from build123d import *

# Parameters (mm, degrees)
SKETCH1_W                                       = 59.1
SKETCH1_H                                       = 59.1
SKETCH1_R                                       = 19.5
SKETCH1_R_2                                     = 1.55
BOSS_EXTRUDE1_DEPTH                             = 4
SKETCH2_W                                       = 59.1
SKETCH2_H                                       = 50
SKETCH2_R                                       = 1.5
BOSS_EXTRUDE2_DEPTH                             = 4
CSK_FOR_M3_FLAT_HEAD_MACHINE_SCREW1_D           = 3.4
CSK_FOR_M3_FLAT_HEAD_MACHINE_SCREW1_CSINK_D     = 6.3
CSK_FOR_M3_FLAT_HEAD_MACHINE_SCREW1_CSINK_ANGLE = 90
CSK_FOR_M4_FLAT_HEAD_MACHINE_SCREW1_D           = 4.5
CSK_FOR_M4_FLAT_HEAD_MACHINE_SCREW1_CSINK_D     = 9.4
CSK_FOR_M4_FLAT_HEAD_MACHINE_SCREW1_CSINK_ANGLE = 90


with BuildPart() as part:
    # Sketch1 → Boss-Extrude1 (new body)
    with BuildSketch(Plane.XY):
        with Locations((23.55, 23.55)):
            Rectangle(SKETCH1_W, SKETCH1_H)
        with Locations((23.55, 23.55)):
            Circle(SKETCH1_R, mode=Mode.SUBTRACT)
        with Locations((0, 47.1)):
            Circle(SKETCH1_R_2, mode=Mode.SUBTRACT)
        with Locations((47.1, 47.1)):
            Circle(SKETCH1_R_2, mode=Mode.SUBTRACT)
        with Locations((47.1, 0)):
            Circle(SKETCH1_R_2, mode=Mode.SUBTRACT)
        Circle(SKETCH1_R_2, mode=Mode.SUBTRACT)
    extrude(amount=BOSS_EXTRUDE1_DEPTH)

    # Sketch2 → Boss-Extrude2 (add)
    with BuildSketch(Plane.XZ.offset(6)):
        with Locations((23.55, -21)):
            Rectangle(SKETCH2_W, SKETCH2_H)
        with Locations(Location((0, -40, 0), (0, 0, 270))):
            Circle(SKETCH2_R, mode=Mode.SUBTRACT)
        with Locations(Location((47.1, -40, 0), (0, 0, 270))):
            Circle(SKETCH2_R, mode=Mode.SUBTRACT)
        with Locations(Location((23.55, -18, 0), (0, 0, 270))):
            Circle(SKETCH2_R, mode=Mode.SUBTRACT)
    extrude(amount=BOSS_EXTRUDE2_DEPTH)

    # CSK for M3 Flat Head Machine Screw1 (through all)
    with Locations(Plane(origin=(0, -6, 0), x_dir=(1, 0, 0), z_dir=(0, 1, 0))):
        with Locations((0, 40), (47.1, 40), (23.55, 18)):
            CounterSinkHole(CSK_FOR_M3_FLAT_HEAD_MACHINE_SCREW1_D / 2, CSK_FOR_M3_FLAT_HEAD_MACHINE_SCREW1_CSINK_D / 2, counter_sink_angle=CSK_FOR_M3_FLAT_HEAD_MACHINE_SCREW1_CSINK_ANGLE)

    # CSK for M4 Flat Head Machine Screw1 (through all)
    with Locations(Plane.XY.offset(4)):
        with Locations((0, 47.1), (47.1, 47.1), (47.1, 0), (0, 0)):
            CounterSinkHole(CSK_FOR_M4_FLAT_HEAD_MACHINE_SCREW1_D / 2, CSK_FOR_M4_FLAT_HEAD_MACHINE_SCREW1_CSINK_D / 2, counter_sink_angle=CSK_FOR_M4_FLAT_HEAD_MACHINE_SCREW1_CSINK_ANGLE)


solid = part.part
Verification items for the finished model (mm, model axes). Coordinates: 2 decimals unless noted, no trailing zeros. Write each loop counter-clockwise with the first axis right and the second up, starting at its lowest first coordinate (ties: lowest second). Pieces come first, ordered by that corner, then holes. Notation, with made-up numbers: M 15.25,60.25 L 48.25,60.25 A16 ccw 48.25,88.25 Z; hole C 34,36.5 d2. An arc over 180 degrees is marked long. Use a Markdown table: item, result.
Q1. Sectioned sample at C-C, the plane z = -18. Record the boundary of the cut face in (x, y), plus the area to 3 significant figures.
Reply:
| item | result |
|---|---|
| outline | M -6,-10 L 21.85,-10 L 21.85,-7.45 L 20.4,-6 L -6,-6 Z; M 25.25,-10 L 53.1,-10 L 53.1,-6 L 26.7,-6 L 25.25,-7.45 Z |
| area | 221 mm² |
Q2. Draft check along X on faces 1 (the face through (23, -6, -23)), 2 (the face through (21.93, -8.74, -18.51)), 3 (the face through (53.1, 8, 1)). Enter one of: +X half, -X half, draft (parallel to the pull), parting line (faces both ways), or undercut.
Reply:
| item | result |
|---|---|
| face 1 | draft |
| face 2 | undercut |
| face 3 | +X half |
Q3. Thickness scan on line 1 (X direction, y = 47, z = 1); line 2 (X direction, y = -7.95, z = -40); line 3 (Y direction, x = 47.1, z = 1.25). Record the ranges inside material, lowest first.
Reply:
| item | result |
|---|---|
| line 1 | x = -6 to -2.25, 2.25 to 44.85, 49.35 to 53.1 |
| line 2 | x = -6 to -1.7, 1.7 to 45.4, 48.8 to 53.1 |
| line 3 | y = -10 to -2.25, 2.25 to 44.85, 49.35 to 53.1 |
Q4. Sectioned sample at D-D, the plane x = 9. Record the boundary of the cut face in (y, z), plus the area to 3 significant figures.
Reply:
| item | result |
|---|---|
| outline | M -10,-46 L -6,-46 L -6,0 L 10.57,0 L 10.57,4 L -10,4 Z; M 36.53,0 L 53.1,0 L 53.1,4 L 36.53,4 Z |
| area | 333 mm² |
Q5. Sectioned sample at A-A, the plane x = 0. Record the boundary of the cut face in (y, z), plus the area to 3 significant figures.
Reply:
| item | result |
|---|---|
| outline | M -10,-46 L -6,-46 L -6,-43.15 L -7.45,-41.7 L -10,-41.7 Z; M -10,-38.3 L -7.45,-38.3 L -6,-36.85 L -6,0 L -2.25,0 L -2.25,1.55 L -4.7,4 L -10,4 Z; M 2.25,0 L 44.85,0 L 44.85,1.55 L 42.4,4 L 4.7,4 L 2.25,1.55 Z; M 49.35,0 L 53.1,0 L 53.1,4 L 51.8,4 L 49.35,1.55 Z |
| area | 373 mm² |
Q6. Sectioned sample at B-B, the plane y = 23.55. Record the boundary of the cut face in (x, z), plus the area to 3 significant figures.
Reply:
| item | result |
|---|---|
| outline | M -6,0 L 4.05,0 L 4.05,4 L -6,4 Z; M 43.05,0 L 53.1,0 L 53.1,4 L 43.05,4 Z |
| area | 80.4 mm² |
Q7. Go/stop test with flat-tipped pins: P1, Ø1.5, axis at x = 6.5, z = -32, coming from the +Y side; P2, Ø5, axis at x = 0, y = 0, coming from the +Z side; P3, Ø5, axis at x = 0, y = 47.1, coming from the -Z side. Record where each tip stops, or that it passes through.
Reply:
| item | result |
|---|---|
| P1 | stops at y = -6 |
| P2 | stops at z = 1.8 |
| P3 | stops at z = 0 |
